Work out the finished part from the listing and answer in its coordinate system (mm). A direction names the side the tool comes from. Coordinates: 2 decimals unless noted, no trailing zeros. Order: outer loops, then holes, each group sorted by start corner. A loop starts at its lowest first (then second) coordinate and runs counter-clockwise, first axis right, second up. Notation, with made-up numbers: (-16, -36) - (36, -36) arc R32 ccw to (36, 0) - close; hole circle Ø11 at (50, 3.5). An arc over 180 degrees is marked (long way). Answer as a JSON object with one key per item and string values. Group by question number.
1) Section D-D (z = 31.5) is taken. Give the vertices of the cut face in (x, y), plus the area to 3 significant figures.
2) Section A-A (y = 8) is taken. Give the vertices of the cut face in (x, z) (3 decimals), plus the area to 3 significant figures.
3) Section C-C (x = -1) is taken. Give the vertices of the cut face in (y, z).
4) Section B-B (z = 22) is taken. Give the vertices of the cut face in (x, y).
5) The mould has two halves that part along X. Classify faces 1 (the face through (7, 11, 28.5)), 2 (the face through (1, 11, 34)), 3 (the face through (-40.972, 32.018, 25.025)): released by +X, released by -X, zero draft, split by the parting line, or undercut.
6) A tool of negligible diameter and unlimited length cuts with its end or side. For faces 4 (the face through (-0.112, 16.691, 1.007)), 5 (the face through (0.37, -7.33, 7.4)), 6 (the face through (-51.19, -11.48, 23.62)), 7 (the face through (-31, -12, 13.58)), 8 (the face through (0, 10, -0.5)), from which of +Z, -Z, +X, -X, +Y, -Y can it reach the whole face along a straight path? Write none if from no direction.
7) Find the intervals of material crossed by line 1 along Y through (x, z) = (-27, 23); line 2 along Z through (x, y) = (-9, 4); line 3 along Z through (x, y) = (-21.5, 31.5), in increasing order.
8) Each of these flat-tipped pins is pushed along its axis until it touches: P1, Ø4, axis at x = 3, y = -6.5, coming from the +Z side; P2, Ø12, axis at x = -1.5, y = 2, coming from the -Z side; P3, Ø1.5, axis at y = 0.5, z = 33.5, coming from the -X side; P4, Ø0.8, axis at x = 12.5, z = -0.5, coming from the -Y side. Where does it stop, or does it pass through?
from build123d import *

# Parameters (mm, degrees)
SKETCH1_W           = 23.83
SKETCH1_H           = 1
BOSS_EXTRUDE1_DEPTH = 20.5
SKETCH2_R           = 1.325
BOSS_EXTRUDE2_DEPTH = 13.75
BOSS_EXTRUDE4_DEPTH = 8
SKETCH5_W           = 21.919818374
SKETCH5_H           = 2.5
BOSS_EXTRUDE5_DEPTH = 50
SKETCH6_R           = 4.25
SKETCH6_R_2         = 1.05
CUT_EXTRUDE1_DEPTH  = 83.099025573
FILLET1_R           = 7
FILLET2_R           = 7
FILLET3_R           = 7
BOSS_EXTRUDE6_START = 41
BOSS_EXTRUDE6_DEPTH = 41


with BuildPart() as part:
    # Sketch1 → Boss-Extrude1 (new body)
    with BuildSketch(Plane(origin=(0, 0, 0), x_dir=(1, 0, 0), z_dir=(0, 1, 0))):
        Rectangle(SKETCH1_W, SKETCH1_H)
    extrude(amount=BOSS_EXTRUDE1_DEPTH)

    # Sketch2 → Boss-Extrude2 (add, symmetric)
    with BuildSketch(Plane(origin=(0, 10.25, 0), x_dir=(1, 0, 0), z_dir=(0, 1, 0))):
        with Locations(Location((-11.915, 0, 0), (0, 0, 270))):
            Circle(SKETCH2_R)
        with Locations(Location((11.915, 0, 0), (0, 0, 270))):
            Circle(SKETCH2_R)
    extrude(amount=BOSS_EXTRUDE2_DEPTH, both=True)

    # Sketch4 → Boss-Extrude4 (add, symmetric)
    with BuildSketch(Plane(origin=(0, 0, 0), x_dir=(0, 0, -1), z_dir=(1, 0, 0))):
        Polygon((-0.5, 16.852307022), (-0.5, 20.5), (-12.5, 33.25), (-35.5, 33.25), (-35.5, 30.75), (-13.580181626, 30.75), align=None)
        Polygon((-0.5, 0), (-0.5, 3.647692978), (-13.580181626, -10.25), (-35.5, -10.25), (-35.5, -12.75), (-12.5, -12.75), align=None)
    extrude(amount=BOSS_EXTRUDE4_DEPTH, both=True)

    # Sketch5 → Boss-Extrude5 (add)
    with BuildSketch(Plane.ZY.offset(8)):
        with Locations((24.540090813, 32)):
            Rectangle(SKETCH5_W, SKETCH5_H)
        with Locations((24.540090813, -11.5)):
            Rectangle(SKETCH5_W, SKETCH5_H)
    extrude(amount=BOSS_EXTRUDE5_DEPTH)

    # Sketch6 → Cut-Extrude1 (cut, through all)
    with BuildSketch(Plane(origin=(0, 33.25, 0), x_dir=(1, 0, 0), z_dir=(0, 1, 0))):
        with Locations(Location((-47.040090813, -24.540090813, 0), (0, 0, 270))):
            Circle(SKETCH6_R)
        with Locations(Location((-54.040090813, -24.540090813, 0), (0, 0, 270))):
            Circle(SKETCH6_R_2)
        with Locations(Location((-47.040090813, -17.540090813, 0), (0, 0, 270))):
            Circle(SKETCH6_R_2)
        with Locations(Location((-40.040090813, -24.540090813, 0), (0, 0, 270))):
            Circle(SKETCH6_R_2)
        with Locations(Location((-47.040090813, -31.540090813, 0), (0, 0, 270))):
            Circle(SKETCH6_R_2)
        with BuildLine():
            ThreePointArc((-58, -24.540090813), (-54.78991692, -16.790264706), (-47.040090813, -13.580181626))
            Line((-47.040090813, -13.580181626), (-58, -13.580181626))
            Line((-58, -13.580181626), (-58, -24.540090813))
        make_face()
        with BuildLine():
            ThreePointArc((-47.040090813, -35.5), (-54.78991692, -32.28991692), (-58, -24.540090813))
            Line((-58, -24.540090813), (-58, -35.5))
            Line((-58, -35.5), (-47.040090813, -35.5))
        make_face()
    extrude(amount=-CUT_EXTRUDE1_DEPTH, mode=Mode.SUBTRACT)

    # Fillet1
    # the kernel refuses this fillet: 7 mm, written as the material it adds along each edge
    with BuildSketch(Plane(origin=(-8, -12.75, 13.580181626), x_dir=(-1, 0, 0), z_dir=(0, 1, 0))) as fillet1_piece_1_section:
        with BuildLine():
            CenterArc((FILLET1_R, -FILLET1_R), FILLET1_R, 90, 90)
            Line((0, -FILLET1_R), (0, 0))
            Line((0, 0), (FILLET1_R, 0))
        make_face()
    fillet1_piece_1 = extrude(amount=2.5, mode=Mode.PRIVATE)
    fillet1_piece_1 = split(fillet1_piece_1, bisect_by=Plane(origin=(-10.020174451, -12.153760937, 11.938833823), z_dir=(0, 0.6853646990049913, 0.7281999926928027)), keep=Keep.TOP, mode=Mode.PRIVATE)
    fillet1_piece_1 = split(fillet1_piece_1, bisect_by=Plane(origin=(-10.020174451, -10.440349189, 13.759333804), z_dir=(0, -0.685364699004991, -0.7281999926928029)), keep=Keep.TOP, mode=Mode.PRIVATE)
    add(fillet1_piece_1)
    with BuildSketch(Plane(origin=(-8, -12.75, 13.580181626), x_dir=(-1, 0, 0), z_dir=(0, 1, 0))) as fillet1_piece_2_section:
        with BuildLine():
            CenterArc((FILLET1_R, -FILLET1_R), FILLET1_R, 90, 90)
            Line((0, -FILLET1_R), (0, 0))
            Line((0, 0), (FILLET1_R, 0))
        make_face()
    fillet1_piece_2 = extrude(amount=20, mode=Mode.PRIVATE)
    fillet1_piece_2 = split(fillet1_piece_2, bisect_by=Plane(origin=(-8.816209607, -9.698679662, 9.628169093), z_dir=(0, 0.6853646990049913, 0.7281999926928027)), keep=Keep.TOP, mode=Mode.PRIVATE)
    fillet1_piece_2 = split(fillet1_piece_2, bisect_by=Plane(origin=(-8.816209607, -10.25, 10.809130305), z_dir=(0, 1, 0)), keep=Keep.TOP, mode=Mode.PRIVATE)
    fillet1_piece_2 = split(fillet1_piece_2, bisect_by=Plane(origin=(-8.816209607, -7.985267914, 11.448669075), z_dir=(0, -0.685364699004991, -0.7281999926928029)), keep=Keep.TOP, mode=Mode.PRIVATE)
    add(fillet1_piece_2)
    with BuildSketch(Plane(origin=(-8, 33.25, 13.580181626), x_dir=(0, 0, -1), z_dir=(0, -1, 0))) as fillet1_piece_3_section:
        with BuildLine():
            CenterArc((FILLET1_R, -FILLET1_R), FILLET1_R, 90, 90)
            Line((0, -FILLET1_R), (0, 0))
            Line((0, 0), (FILLET1_R, 0))
        make_face()
    fillet1_piece_3 = extrude(amount=2.5, mode=Mode.PRIVATE)
    fillet1_piece_3 = split(fillet1_piece_3, bisect_by=Plane(origin=(-10.020174451, 32.653760936, 11.938833823), z_dir=(0, -0.6853646990049912, 0.7281999926928028)), keep=Keep.TOP, mode=Mode.PRIVATE)
    fillet1_piece_3 = split(fillet1_piece_3, bisect_by=Plane(origin=(-10.020174451, 30.940349189, 13.759333804), z_dir=(0, 0.6853646990049909, -0.7281999926928031)), keep=Keep.TOP, mode=Mode.PRIVATE)
    add(fillet1_piece_3)
    with BuildSketch(Plane(origin=(-8, 33.25, 13.580181626), x_dir=(0, 0, -1), z_dir=(0, -1, 0))) as fillet1_piece_4_section:
        with BuildLine():
            CenterArc((FILLET1_R, -FILLET1_R), FILLET1_R, 90, 90)
            Line((0, -FILLET1_R), (0, 0))
            Line((0, 0), (FILLET1_R, 0))
        make_face()
    fillet1_piece_4 = extrude(amount=20, mode=Mode.PRIVATE)
    fillet1_piece_4 = split(fillet1_piece_4, bisect_by=Plane(origin=(-8.816209616, 30.198679665, 9.628169097), z_dir=(0, -0.6853646990049912, 0.7281999926928028)), keep=Keep.TOP, mode=Mode.PRIVATE)
    fillet1_piece_4 = split(fillet1_piece_4, bisect_by=Plane(origin=(-8.816209616, 28.485267918, 11.448669078), z_dir=(0, 0.6853646990049909, -0.7281999926928031)), keep=Keep.TOP, mode=Mode.PRIVATE)
    fillet1_piece_4 = split(fillet1_piece_4, bisect_by=Plane(origin=(-8.816209616, 30.75, 10.809130308), z_dir=(0, -1, 0)), keep=Keep.TOP, mode=Mode.PRIVATE)
    add(fillet1_piece_4)
    # the kernel refuses this fillet: 7 mm, written as the material it takes off along each edge
    with BuildSketch(Plane(origin=(8, 7.25, 35.5), x_dir=(0, 0, -1), z_dir=(0, -1, 0))) as fillet1_2_piece_1:
        with BuildLine():
            CenterArc((FILLET1_R, -FILLET1_R), FILLET1_R, 90, 90)
            Line((0, -FILLET1_R), (0, 0))
            Line((0, 0), (FILLET1_R, 0))
        make_face()
    extrude(amount=37.5, mode=Mode.SUBTRACT)
    with BuildSketch(Plane(origin=(8, 50.75, 35.5), x_dir=(-1, 0, 0), z_dir=(0, -1, 0))) as fillet1_2_piece_2:
        with BuildLine():
            CenterArc((FILLET1_R, FILLET1_R), FILLET1_R, 180, 90)
            Line((0, FILLET1_R), (0, 0))
            Line((0, 0), (FILLET1_R, 0))
        make_face()
    extrude(amount=37.5, mode=Mode.SUBTRACT)

    # Fillet2
    fillet2_edges = [part.edges().sort_by_distance(p)[0] for p in [
        (0, 16.852307022, 0.5),
        (0, 3.647692978, 0.5),
    ]]
    fillet(fillet2_edges, radius=FILLET2_R)

    # Fillet3
    # the kernel refuses this fillet: 7 mm, written as the material it adds along each edge
    with BuildSketch(Plane(origin=(-8, 20.5, 0.5), x_dir=(0, 0.7281999926925888, 0.6853646990052185), z_dir=(1, 0, 0))) as fillet3_piece_1:
        with BuildLine():
            CenterArc((2.423417163, -7), FILLET3_R, 90, 26.366519243)
            Line((-0.685364699, -0.728199993), (0, 0))
            Line((0, 0), (2.423417163, 0))
        make_face()
    extrude(amount=16)
    with BuildSketch(Plane(origin=(8, 0, 0.5), x_dir=(0, 0, -1), z_dir=(-1, 0, 0))) as fillet3_piece_2:
        with BuildLine():
            CenterArc((3.436475374, 6.562285254), FILLET3_R, 223.264295411, 26.366519243)
            Line((-1.660924575, 1.764732361), (0, 0))
            Line((0, 0), (1, 0))
        make_face()
    extrude(amount=16)

    # Sketch8 → Boss-Extrude6 (add)
    with BuildSketch(Plane(origin=(0, -10.25, 0), x_dir=(1, 0, 0), z_dir=(0, 1, 0)).offset(BOSS_EXTRUDE6_START)):
        with BuildLine():
            ThreePointArc((1, -35.5), (5.949747468, -33.449747468), (8, -28.5))
            Line((8, -28.5), (5, -28.5))
            ThreePointArc((5, -28.5), (3.422054899, -30.922054899), (1, -32.5))
            Line((1, -32.5), (1, -35.5))
        make_face()
    extrude(amount=-BOSS_EXTRUDE6_DEPTH)


solid = part.part
Report:
{
 "1": {"outline": "(-55.51, -12.75) - (-48.09, -12.75) - (-48.09, -10.25) - (-55.51, -10.25) - close; (-55.51, 30.75) - (-48.09, 30.75) - (-48.09, 33.25) - (-55.51, 33.25) - close; (-45.99, -12.75) - (7.32, -12.75) - (7.32, 33.25) - (-45.99, 33.25) - (-45.99, 30.75) - (2.77, 30.75) - (2.77, -10.25) - (-45.99, -10.25) - close", "area": "491 mm²"},
 "2": {"outline": "(-10.688, -0.5) - (10.688, -0.5) arc R1.325 ccw (long way) to (10.688, 0.5) - (-10.688, 0.5) arc R1.325 ccw (long way) to start; (1, 32.5) arc R7 cw to (5, 28.5) - (8, 28.5) arc R7 ccw to (1, 35.5) - close", "area": "60.5 mm²"},
 "3": {"outline": "(-12.75, 12.5) - (-1.76, 2.16) arc R7 cw to (0, -0.5) - (20.5, -0.5) arc R7 cw to (22.26, 2.16) - (33.25, 12.5) - (33.25, 35.5) - (30.75, 35.5) - (30.75, 13.58) - (18.87, 2.4) arc R7 cw to (14.08, 0.5) - (6.42, 0.5) arc R7 cw to (1.63, 2.4) - (-10.25, 13.58) - (-10.25, 35.5) - (-12.75, 35.5) - close"},
 "4": {"outline": "(-57.7, -12.75) - (-50.45, -12.75) - (-50.45, -10.25) - (-57.7, -10.25) - close; (-57.7, 30.75) - (-50.45, 30.75) - (-50.45, 33.25) - (-57.7, 33.25) - close; (-43.63, -12.75) - (8, -12.75) - (8, -10.25) - (-43.63, -10.25) - close; (-43.63, 30.75) - (8, 30.75) - (8, 33.25) - (-43.63, 33.25) - close"},
 "5": {"face 1": "zero draft", "face 2": "released by -X", "face 3": "undercut"},
 "6": {"face 4": "none", "face 5": "-Z, +X, -X, -Y", "face 6": "+Y, -Y", "face 7": "-Z, -X, +Y, -Y", "face 8": "-Z, +Y, -Y"},
 "7": {"line 1": "y = -12.75 to -10.25, 30.75 to 33.25", "line 2": "z = -0.5 to 0.5", "line 3": "z = 13.58 to 35.5"},
 "8": {"P1": "stops at z = 35.5", "P2": "stops at z = -0.5", "P3": "stops at x = 1", "P4": "stops at y = -3.5"}
}
